Check sheet for the modelled part. Datum: model origin and axes. Units: mm. A direction names the side the tool comes from. Round coordinates to 2 decimals unless told otherwise and drop trailing zeros. Write each loop counter-clockwise with the first axis right and the second up, starting at its lowest first coordinate (ties: lowest second). Pieces come first, ordered by that corner, then holes. Notation, with made-up numbers: M 38,51 L 80,51 A33 ccw 80,83 Z; hole C 6.5,-31 d8. An arc over 180 degrees is marked long. One line per item, written item: value.
from build123d import *

# Parameters (mm, degrees)
CYLINDER032_R     = 1.75
CYLINDER032_DEPTH = 8
CYLINDER035_R     = 1.75
CYLINDER035_DEPTH = 8
CYLINDER038_R     = 1.6
CYLINDER038_DEPTH = 8
CYLINDER039_R     = 1.6
CYLINDER039_DEPTH = 8
CYLINDER037_W     = 7
CYLINDER037_H     = 8
CYLINDER037_ANGLE = 90
BOX025_W          = 78
BOX025_H          = 3
BOX025_DEPTH      = 7
BOX026_W          = 40
BOX026_H          = 3
BOX026_DEPTH      = 7
CYLINDER034_R     = 3.5
CYLINDER034_DEPTH = 8
CYLINDER031_R     = 3.5
CYLINDER031_DEPTH = 8
BOX027_W          = 40
BOX027_H          = 3
BOX027_DEPTH      = 7
CYLINDER036_W     = 7
CYLINDER036_H     = 8
CYLINDER036_ANGLE = 90


with BuildPart() as cuts:
    # Cylinder032 → Cylinder032 (new body)
    with BuildSketch(Plane(origin=(13.5, -2, 61.5), x_dir=(1, 0, 0), z_dir=(0, -1, 0))):
        Circle(CYLINDER032_R)
    extrude(amount=CYLINDER032_DEPTH)


with BuildPart() as cuts001:
    # Cylinder035 → Cylinder035 (new body)
    with BuildSketch(Plane(origin=(62.5, -2, 61.5), x_dir=(1, 0, 0), z_dir=(0, -1, 0))):
        Circle(CYLINDER035_R)
    extrude(amount=CYLINDER035_DEPTH)


with BuildPart() as m3screw:
    # Cylinder038 → Cylinder038 (new body)
    with BuildSketch(Plane(origin=(75.5, -2, 100.5), x_dir=(1, 0, 0), z_dir=(0, -1, 0))):
        Circle(CYLINDER038_R)
    extrude(amount=CYLINDER038_DEPTH)


with BuildPart() as c4oldcuts:
    # Cylinder039 → Cylinder039 (new body)
    with BuildSketch(Plane(origin=(2.5, -2, 100.5), x_dir=(1, 0, 0), z_dir=(0, -1, 0))):
        Circle(CYLINDER039_R)
    extrude(amount=CYLINDER039_DEPTH)

    # Fusion016: union cuts, cuts001, m3Screw
    add(cuts.part)
    add(cuts001.part)
    add(m3screw.part)


with BuildPart() as cylinder037:
    # Cylinder037 → Cylinder037 (revolve)
    with BuildSketch(Plane(origin=(0, -2, 98), x_dir=(1, 0, 0), z_dir=(0, 0, -1))):
        with Locations((3.5, 4)):
            Rectangle(CYLINDER037_W, CYLINDER037_H)
    revolve(axis=Axis((0, -2, 98), (0, -1, 0)), revolution_arc=CYLINDER037_ANGLE)


with BuildPart() as cube020:
    # Box025 → Box025 (new body)
    with BuildSketch(Plane(origin=(0, -5, 58), x_dir=(1, 0, 0), z_dir=(0, 0, 1))):
        with Locations((39, 1.5)):
            Rectangle(BOX025_W, BOX025_H)
    extrude(amount=BOX025_DEPTH)


with BuildPart() as cube021:
    # Box026 → Box026 (new body)
    with BuildSketch(Plane(origin=(7, -5, 58), x_dir=(0, 0, 1), z_dir=(-1, 0, 0))):
        with Locations((20, 1.5)):
            Rectangle(BOX026_W, BOX026_H)
    extrude(amount=BOX026_DEPTH)


with BuildPart() as cylinder034:
    # Cylinder034 → Cylinder034 (new body)
    with BuildSketch(Plane(origin=(62.5, -2, 61.5), x_dir=(1, 0, 0), z_dir=(0, -1, 0))):
        Circle(CYLINDER034_R)
    extrude(amount=CYLINDER034_DEPTH)


with BuildPart() as cylinder031:
    # Cylinder031 → Cylinder031 (new body)
    with BuildSketch(Plane(origin=(13.5, -2, 61.5), x_dir=(1, 0, 0), z_dir=(0, -1, 0))):
        Circle(CYLINDER031_R)
    extrude(amount=CYLINDER031_DEPTH)


with BuildPart() as fusion014:
    # Box027 → Box027 (new body)
    with BuildSketch(Plane(origin=(78, -5, 58), x_dir=(0, 0, 1), z_dir=(-1, 0, 0))):
        with Locations((20, 1.5)):
            Rectangle(BOX027_W, BOX027_H)
    extrude(amount=BOX027_DEPTH)

    # Fusion014: union Cube020, Cube021, Cylinder034, Cylinder031
    add(cube020.part)
    add(cube021.part)
    add(cylinder034.part)
    add(cylinder031.part)


with BuildPart() as c4hold001:
    # Cylinder036 → Cylinder036 (revolve)
    with BuildSketch(Plane(origin=(78, -2, 98), x_dir=(0, 0, 1), z_dir=(1, 0, 0))):
        with Locations((3.5, 4)):
            Rectangle(CYLINDER036_W, CYLINDER036_H)
    revolve(axis=Axis((78, -2, 98), (0, -1, 0)), revolution_arc=CYLINDER036_ANGLE)

    # Fusion015: union Cylinder037, Fusion014
    add(cylinder037.part)
    add(fusion014.part)

    # Cut024: cut c4oldCuts
    add(c4oldcuts.part, mode=Mode.SUBTRACT)


solid = c4hold001.part
Q1. Sectioned sample at D-D on z = 61.5. Enter the section's corners in (x, y), and give its area (3 significant figures).
Completed:
outline: M 0,-5 L 10,-5 L 10,-10 L 11.75,-10 L 11.75,-2 L 0,-2 Z; M 15.25,-10 L 17,-10 L 17,-5 L 59,-5 L 59,-10 L 60.75,-10 L 60.75,-2 L 15.25,-2 Z; M 64.25,-10 L 66,-10 L 66,-5 L 78,-5 L 78,-2 L 64.25,-2 Z
area: 248 mm^2
Q2. Scan lines: line 1 (X direction, y = -2.75, z = 87); line 2 (Z direction, x = 16.5, y = -2.5); line 3 (Y direction, x = 73, z = 61.5). Record each from-to range of solid material in increasing order. Write a range as [from, to].
Completed:
line 1: [0, 7], [71, 78]
line 2: [58, 65]
line 3: [-5, -2]
Q3. Sectioned sample at A-A on y = -8. Enter the section's corners in (x, z), and give its area (3 significant figures).
Completed:
outline: M 0,98 L 7,98 A7 ccw 0,105 Z; C 13.5,61.5 d7; C 62.5,61.5 d7; M 71,98 L 78,98 L 78,105 A7 ccw Z; hole C 2.5,100.5 d3.2; hole C 13.5,61.5 d3.5; hole C 62.5,61.5 d3.5; hole C 75.5,100.5 d3.2
area: 119 mm^2
Q4. Depth check by flat-ended pin: P1, Ø8, axis at x = 71.5, z = 82, coming from the -Y side; P2, Ø4, axis at x = 75.5, y = -8.5, coming from the -Z side; P3, Ø2.5, axis at x = 33.5, y = -3, coming from the +Z side. Enter the tip coordinate at first touch or a pass-through.
Completed:
P1: y = -5
P2: z = 98
P3: z = 65
Q5. Sectioned sample at C-C on y = -3.5. Enter the section's corners in (x, z), and give its area (3 significant figures).
Completed:
outline: M 0,58 L 78,58 L 78,105 A7 ccw 71,98 L 71,65 L 7,65 L 7,98 A7 ccw 0,105 Z; hole C 2.5,100.5 d3.2; hole C 13.5,61.5 d3.5; hole C 62.5,61.5 d3.5; hole C 75.5,100.5 d3.2
area: 1,050 mm^2
Q6. Sectioned sample at B-B on z = 89.5. Enter the section's corners in (x, y), and give its area (3 significant figures).
Completed:
outline: M 0,-5 L 7,-5 L 7,-2 L 0,-2 Z; M 71,-5 L 78,-5 L 78,-2 L 71,-2 Z
area: 42.0 mm^2
Q7. Draft check along Z on faces 1 (the flat face through (4, -10, 102)), 2 (the cylindrical face through (64.117, -5.944, 60.83)), 3 (the cylindrical face through (59.003, -7.465, 61.654)). Enter one of: pulls with the +Z half, pulls with the -Z half, needs draft (parallel to the pull), parting line crosses it, or undercut.
Completed:
face 1: needs draft
face 2: undercut
face 3: parting line crosses it
Q8. Access from +Z, -Z, +X, -X, +Y, -Y to the whole of each face (thin tool, end or side, straight path). Record for faces 4 (the cylindrical face through (2.292, -5.944, 102.086)), 5 (the flat face through (39, -3, 65)), 6 (the flat face through (3, -8, 98)), 7 (the flat face through (38, -3, 58)), 8 (the cylindrical face through (15.115, -7.465, 58.395)).
Completed:
face 4: +Y, -Y
face 5: +Z, +Y, -Y
face 6: -Z, +X, -X, -Y
face 7: -Z, +X, -X, +Y, -Y
face 8: -Y
